Autodesk Inventor part; units mm, degrees
ref_plane "YZ Plane" through (0, 0, 0) normal (1, 0, 0) x (0, 1, 0)
ref_plane "XZ Plane" through (0, 0, 0) normal (0, 1, 0) x (-1, 0, 0)
ref_plane "XY Plane" through (0, 0, 0) normal (0, 0, 1) x (1, 0, 0)
sketch "Sketch1" plane through (0, 0, 0) normal (0, 0, 1) x (1, 0, 0)
  circle A0 centre (0, 0) radius 75
  circle A1 centre (0, 0) radius 140
  dimension "d22" = 150
  dimension "d23" = 280
extrude "Plate1" add sketch "Sketch1" along normal blind 10
sketch "Sketch5" plane through (0, 0, 10) normal (0, 0, 1) x (1, 0, 0)
  circle A0 centre (0, 120) radius 11
  circle A1 centre (0, 0) radius 120 construction
  dimension "d25" = 240
  dimension "d24" = 22
extrude "Cut1" cut sketch "Sketch5" against normal blind 10
pattern_circular "Circular Pattern1" count 8 over 360 about axis through (0, 0, 0) along (0, 0, 1) of "Cut1"
equation "\"d26\" = Thickness"
equation "\"d2\" = Thickness"
equation "\"BendReliefDepth\" = 0.5 * Thickness"
equation "\"TransitionRadius\" = BendRadius"
equation "\"JacobiRadiusSize\" = BendRadius"
properties part number "Main filter Flange" material "Stainless Steel"
Verification items for the finished model (mm, model axes). Round coordinates to 2 decimals unless told otherwise and drop trailing zeros. Loops run counter-clockwise (first coordinate to the right, second up) from the corner with the lowest first, then second, coordinate; pieces in that order, holes last. Notation, with made-up numbers: (-34, 76.5) - (17, 76.5) arc R19 cw to (17, 87.5) - close; hole circle Ø1 at (6.5, 89). An arc over 180 degrees is marked (long way). Use one line per item in the form item = value.
1. Draft check along X on faces 1 (the cylindrical face through (-92.965, 77.424, 5.07)), 2 (the flat face through (60, -60, 10)), 3 (the cylindrical face through (-111.1, 85.19, 4.93)), 4 (the cylindrical face through (130.906, 1.432, 5.07)). Enter one of: pulls with the +X half, pulls with the -X half, needs draft (parallel to the pull), parting line crosses it, or undercut.
A:
face_1 = undercut
face_2 = needs draft
face_3 = parting line crosses it
face_4 = undercut
2. Scan lines: probe 1 along Y at (x, z) = (0, 2.5); probe 2 along Y at (x, z) = (-78, 9); probe 3 along Y at (x, z) = (-78.5, 4.75). Record each from-to range of solid material in increasing order.
A:
probe_1 = -140 to -131, -109 to -75, 75 to 109, 131 to 140
probe_2 = -116.26 to -93.46, -76.25 to 76.25, 93.46 to 116.26
probe_3 = -115.92 to -93.83, -75.87 to 75.87, 93.83 to 115.92
3. Section check C-C on x = -120. Record the cut outline in (y, z).
A:
outline = (-72.11, 0) - (-11, 0) - (-11, 10) - (-72.11, 10) - close; (11, 0) - (72.11, 0) - (72.11, 10) - (11, 10) - close
4. Section check A-A on x = 0. Record the cut outline in (y, z).
A:
outline = (-140, 0) - (-131, 0) - (-131, 10) - (-140, 10) - close; (-109, 0) - (-75, 0) - (-75, 10) - (-109, 10) - close; (75, 0) - (109, 0) - (109, 10) - (75, 10) - close; (131, 0) - (140, 0) - (140, 10) - (131, 10) - close
5. Section check B-B on y = -63.5. Record the cut outline in (x, z).
A:
outline = (-124.77, 0) - (-39.91, 0) - (-39.91, 10) - (-124.77, 10) - close; (39.91, 0) - (124.77, 0) - (124.77, 10) - (39.91, 10) - close
6. Gauge pin test, flat ends, axial feed: pin 1 Ø20 at (x, y) = (-84.85, 84.85) entering from -Z; pin 2 Ø1.5 at (x, z) = (70, 3.5) entering from +Y; pin 3 Ø5 at (y, z) = (-80.5, 6) entering from -X; pin 4 Ø1.5 at (y, z) = (-46, 7.5) entering from -X. Record the tip position at first contact, or that the pin passes through.
A:
pin_1 = through
pin_2 = 121.67
pin_3 = -116.26
pin_4 = -132.49
